```python
from build123d import *

# Parameters (mm, degrees)
CUT_EXTRUDE1_REACH             = 23.896
SKETCH2_R                      = 1
CUT_EXTRUDE1_DIRECTION_2_REACH = 23.896


with BuildPart() as part:
    # Sketch1 → Revolve1 (revolve)
    with BuildSketch(Plane.XY, mode=Mode.PRIVATE) as revolve1_sk:
        with BuildLine():
            Line((3.5, 8.5), (3.5, 0))
            Line((3.5, 0), (11.85, 0))
            Line((11.85, 0), (12.587068007, 0.737068007))
            ThreePointArc((12.587068007, 0.737068007), (10.5, 4.25), (12.587068007, 7.762931993))
            Line((12.587068007, 7.762931993), (11.85, 8.5))
            Line((11.85, 8.5), (6.75, 8.5))
            ThreePointArc((6.75, 8.5), (5.866116524, 8.866116524), (5.5, 9.75))
            Line((5.5, 9.75), (5.5, 12.75))
            Line((5.5, 12.75), (3.5, 12.75))
            Line((3.5, 12.75), (3.5, 8.5))
        make_face()
    revolve(revolve1_sk.sketch.rotate(Axis((0, 0, 0), (0, 1, 0)), 90), axis=Axis((0, 0, 0), (0, 1, 0)))

    # Sketch2 → Cut-Extrude1 (cut, up to next)
    with BuildSketch(Plane.XY, mode=Mode.PRIVATE) as cut_extrude1_sk1:
        with Locations((0, 9.75)):
            Circle(SKETCH2_R)
    cut_extrude1_tool1 = extrude(cut_extrude1_sk1.sketch, amount=-CUT_EXTRUDE1_REACH, mode=Mode.PRIVATE) & part.part
    add(cut_extrude1_tool1.solids().sort_by_distance((0, 9.75, 0))[0], mode=Mode.SUBTRACT)

    # Sketch2 → Cut-Extrude1 direction 2 (cut, up to next)
    with BuildSketch(Plane.XY, mode=Mode.PRIVATE) as cut_extrude1_direction_2_sk1:
        with Locations((0, 9.75)):
            Circle(SKETCH2_R)
    cut_extrude1_direction_2_tool1 = extrude(cut_extrude1_direction_2_sk1.sketch, amount=CUT_EXTRUDE1_DIRECTION_2_REACH, mode=Mode.PRIVATE) & part.part
    add(cut_extrude1_direction_2_tool1.solids().sort_by_distance((0, 9.75, 0))[0], mode=Mode.SUBTRACT)


solid = part.part
```
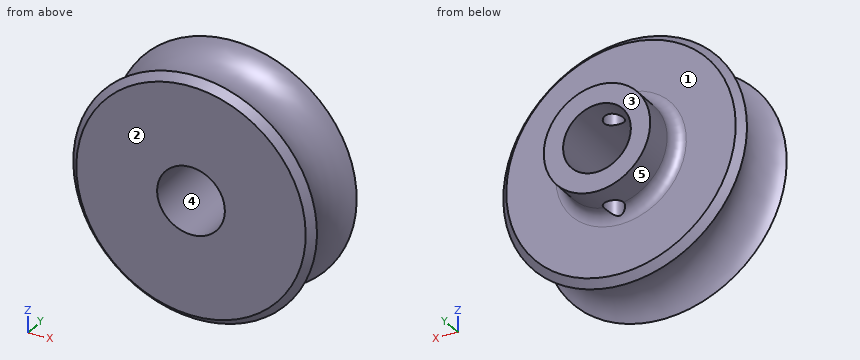
Part model, mm, in its own coordinate system. Face numbers are marked on the shaded views. A direction names the side the tool comes from. Coordinates: 2 decimals unless noted, no trailing zeros. Loops run counter-clockwise (first coordinate to the right, second up) from the corner with the lowest first, then second, coordinate; pieces in that order, holes last. Notation, with made-up numbers: (54.5, -16.75) - (77.5, -16.75) arc R17 ccw to (77.5, 4.25) - close; hole circle Ø7 at (13.25, 65.5). An arc over 180 degrees is marked (long way). Write item = value, one per line. Start each with the question number.
Item 1: Cut at B-B, the plane z = 0. Give the cut face in (x, y).
Item 2: Flat gauge pins, fed straight in: pin 1 Ø1.6 at (x, y) = (0, 9.75) entering from -Z (3 decimals); pin 2 Ø1.5 at (x, y) = (-2, 11) entering from +Z; pin 3 Ø3 at (y, z) = (9, 7.5) entering from +X; pin 4 Ø2 at (x, z) = (4.5, 5.5) entering from +Y. Where does each tip first touch, or does it go through?
Item 3: Mould opens along X. For the marked faces 3, 4 and 5 say: released by +X, released by -X, zero draft, split by the parting line, or undercut.
Item 4: 3-axis set-ups, long thin cutter, end or side, ignore diameter. For the marked faces 1 and 2: which of +Z, -Z, +X, -X, +Y, -Y reach the whole face in a straight line?
Item 5: Cut at A-A, the plane x = 0. Give the cut face in (y, z).
Item 6: Cut at C-C, the plane y = 1.5. Give the cut face in (x, z), and give its area (3 significant figures).
Item 7: Wall check: L1, parallel to Y at x = 0, z = 4.9; L2, parallel to Y at x = 8.25, z = -1; L3, parallel to Z at x = -1.5, y = 11.5. Give the ranges that are in metal, low to high. Write a range as from..to.
The answers:
q1.outline = (-12.59, 0.74) - (-11.85, 0) - (-3.5, 0) - (-3.5, 12.75) - (-5.5, 12.75) - (-5.5, 9.75) arc R1.25 cw to (-6.75, 8.5) - (-11.85, 8.5) - (-12.59, 7.76) arc R4 cw to start; (3.5, 0) - (11.85, 0) - (12.59, 0.74) arc R4 cw to (12.59, 7.76) - (11.85, 8.5) - (6.75, 8.5) arc R1.25 cw to (5.5, 9.75) - (5.5, 12.75) - (3.5, 12.75) - close
q2.pin_1 = through
q2.pin_2 = 5.36
q2.pin_3 = 10.69
q2.pin_4 = 8.68
q3.face_3 = zero draft
q3.face_4 = undercut
q3.face_5 = split by the parting line
q4.face_1 = +Y
q4.face_2 = +Z, -Z, +X, -X, -Y
q5.outline = (0, -11.85) - (0.74, -12.59) arc R4 cw to (7.76, -12.59) - (8.5, -11.85) - (8.5, -6.75) arc R1.25 cw to (8.75, -6) - (8.75, -3.5) - (0, -3.5) - close; (0, 3.5) - (8.75, 3.5) - (8.75, 6) arc R1.25 cw to (8.5, 6.75) - (8.5, 11.85) - (7.76, 12.59) arc R4 cw to (0.74, 12.59) - (0, 11.85) - close; (10.75, -5.5) - (12.75, -5.5) - (12.75, -3.5) - (10.75, -3.5) - close; (10.75, 3.5) - (12.75, 3.5) - (12.75, 5.5) - (10.75, 5.5) - close
q6.outline = circle Ø23.19 at (0, 0); hole circle Ø7 at (0, 0)
q6.area = 384 mm2
q7.L1 = 0..8.75, 10.75..12.75
q7.L2 = 0..8.5
q7.L3 = -5.29..-3.16, 3.16..5.29
